from build123d import *

# Parameters (mm, degrees)
SKETCH_1_W          = 22
SKETCH_1_H          = 19
EXTRUDE_1_DEPTH     = 1
SKETCH_2_W          = 18
SKETCH_2_H          = 18
EXTRUDE_2_DEPTH     = 2
CUT_EXTRUDE_1_DEPTH = 4


with BuildPart() as part:
    # Эскиз1 → Бобышка-Вытянуть1 (new body)
    with BuildSketch(Plane.XY):
        Rectangle(SKETCH_1_W, SKETCH_1_H)
    extrude(amount=EXTRUDE_1_DEPTH)

    # Эскиз2 → Бобышка-Вытянуть2 (add)
    with BuildSketch(Plane.XY.offset(1)):
        Rectangle(SKETCH_2_W, SKETCH_2_H)
    extrude(amount=EXTRUDE_2_DEPTH)

    # Эскиз3 → Вырез-Вытянуть1 (cut, through all)
    with BuildSketch(Plane.XY.offset(3)):
        with BuildLine():
            Line((-11, -4.2), (-11, -5.8))
            ThreePointArc((-11, -5.8), (-10.2, -5), (-11, -4.2))
        make_face()
        with BuildLine():
            Line((-11, -1.63), (-11, -3.23))
            ThreePointArc((-11, -3.23), (-10.2, -2.43), (-11, -1.63))
        make_face()
        with BuildLine():
            Line((-11, 0.94), (-11, -0.66))
            ThreePointArc((-11, -0.66), (-10.2, 0.14), (-11, 0.94))
        make_face()
        with BuildLine():
            Line((-11, 3.51), (-11, 1.91))
            ThreePointArc((-11, 1.91), (-10.2, 2.71), (-11, 3.51))
        make_face()
        with BuildLine():
            Line((-11, 6.08), (-11, 4.48))
            ThreePointArc((-11, 4.48), (-10.2, 5.28), (-11, 6.08))
        make_face()
        with BuildLine():
            Line((11, -4.2), (11, -5.8))
            ThreePointArc((11, -5.8), (10.2, -5), (11, -4.2))
        make_face()
        with BuildLine():
            Line((11, -1.63), (11, -3.23))
            ThreePointArc((11, -3.23), (10.2, -2.43), (11, -1.63))
        make_face()
        with BuildLine():
            Line((11, 0.94), (11, -0.66))
            ThreePointArc((11, -0.66), (10.2, 0.14), (11, 0.94))
        make_face()
        with BuildLine():
            Line((11, 3.51), (11, 1.91))
            ThreePointArc((11, 1.91), (10.2, 2.71), (11, 3.51))
        make_face()
        with BuildLine():
            Line((11, 6.08), (11, 4.48))
            ThreePointArc((11, 4.48), (10.2, 5.28), (11, 6.08))
        make_face()
        with BuildLine():
            Line((11, 8.65), (11, 7.05))
            ThreePointArc((11, 7.05), (10.2, 7.85), (11, 8.65))
        make_face()
    extrude(amount=-CUT_EXTRUDE_1_DEPTH, mode=Mode.SUBTRACT)


solid = part.part
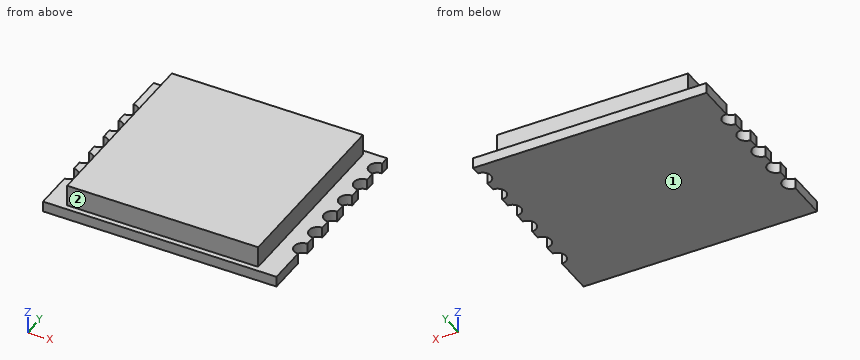
The listing builds one solid part. Answer for the finished solid, in the listing's coordinates (mm). Face numbers are marked on the shaded views. A direction names the side the tool comes from. Coordinates: 2 decimals unless noted, no trailing zeros. Loops run counter-clockwise (first coordinate to the right, second up) from the corner with the lowest first, then second, coordinate; pieces in that order, holes last.
1) Find section A-A on y = -2.43. Write down the section's boundary in (x, z).
2) Find section C-C on z = 0.4. Write down the section's boundary in (x, y), then the cut area to 3 significant figures.
3) A tool of negligible diameter and unlimited length cuts with its end or side. For the marked faces 1 and 2, from which of +Z, -Z, +X, -X, +Y, -Y can it reach the whole face along a straight path? Write none if from no direction.
4) Find the intervals of material crossed by L1, parallel to X at y = -5.5, z = 1.4; L2, parallel to X at y = 7.5, z = 0.95, in increasing order.
5) Find section B-B on x = 0. Write down the section's boundary in (y, z), then the cut area to 3 significant figures.
6) Flat-ended cylindrical pins translate along their axes: pin 1 Ø1.6 at (x, z) = (0.5, 2) entering from +Y; pin 2 Ø1 at (y, z) = (-2.5, 2.5) entering from +X. Find the tip coordinate at first contact, or state that the pin passes through.
7) Find section D-D on z = 2.75. Write down the section's boundary in (x, y).
Values:
1. outline: (-10.2, 0) - (10.2, 0) - (10.2, 1) - (9, 1) - (9, 3) - (-9, 3) - (-9, 1) - (-10.2, 1) - close
2. outline: (-11, -9.5) - (11, -9.5) - (11, -5.8) arc R0.8 cw to (11, -4.2) - (11, -3.23) arc R0.8 cw to (11, -1.63) - (11, -0.66) arc R0.8 cw to (11, 0.94) - (11, 1.91) arc R0.8 cw to (11, 3.51) - (11, 4.48) arc R0.8 cw to (11, 6.08) - (11, 7.05) arc R0.8 cw to (11, 8.65) - (11, 9.5) - (-11, 9.5) - (-11, 6.08) arc R0.8 cw to (-11, 4.48) - (-11, 3.51) arc R0.8 cw to (-11, 1.91) - (-11, 0.94) arc R0.8 cw to (-11, -0.66) - (-11, -1.63) arc R0.8 cw to (-11, -3.23) - (-11, -4.2) arc R0.8 cw to (-11, -5.8) - close
2. area: 407 mm2
3. face 1: -Z, +X, -X, +Y, -Y
3. face 2: +Z, +X, -X, -Y
4. L1: x = -9 to 9
4. L2: x = -11 to 10.28
5. outline: (-9.5, 0) - (9.5, 0) - (9.5, 1) - (9, 1) - (9, 3) - (-9, 3) - (-9, 1) - (-9.5, 1) - close
5. area: 55.0 mm2
6. pin 1: stops at y = 9
6. pin 2: stops at x = 9
7. outline: (-9, -9) - (9, -9) - (9, 9) - (-9, 9) - close
